Here's how the part is built. I have some questions about the finished solid (model axes, mm). A direction names the side the tool comes from. Coordinates: 2 decimals unless noted, no trailing zeros. Loops run counter-clockwise (first coordinate to the right, second up) from the corner with the lowest first, then second, coordinate; pieces in that order, holes last. Notation, with made-up numbers: M -11.75,41 L 9.25,41 A22 ccw 9.25,63 Z; hole C 54.5,-32 d8. An arc over 180 degrees is marked long. Use CSV: the item, a comma, the result in double quotes. Start each with the question number.
Q1. If we section it at D-D (z = 158.5): Please give me the cut outline in (x, y), and give its area (3 significant figures).
Q2. Please list where these lines run through material, in increasing order: probe 1 along Z at (x, y) = (193.5, -2.7); probe 2 along Z at (x, y) = (209, -2.05); probe 3 along Z at (x, y) = (421, -2.3). Write a range as [from, to].
Q3. If we section it at A-A (x = 37): Please give me the cut outline in (y, z).
Q4. If we section it at B-B (y = -2.35): State how many separate pieces and enclosed holes the cut face has, and give its area (3 significant figures).
Q5. Which directions (+Z, -Z, +X, -X, +Y, -Y) give clear straight access to the entire face, cutting with the end or side of a thin tool? Please do faces 5 (the flat face through (-7, 0, 118)), 6 (the cylindrical face through (-185.198, -1.479, -390.683)).
Q6. For pin 1 Ø0.9 at (x, y) = (429.5, -2) entering from +Z; pin 2 Ø0.5 at (x, y) = (-166.5, -1) entering from +Z; pin 3 Ø0.9 at (y, z) = (-1, 101.5) entering from +X, each with a flat end and sliding along its axis, tell me the tip position at first contact or that it passes through.
Q7. If we mould it in two halves opening along X, with no side actions, what happens to faces 1 (the cylindrical face through (-499.516, -1.479, 21.984)), 2 (the flat face through (-7, -3, 118)), 3 (the flat face through (-45.813, -1.479, 2.98)), 4 (the flat face through (356.448, -1.479, -3.983))? For each: +X half, -X half, draft (parallel to the pull), parting line (faces both ways), or undercut.
from build123d import *

# Parameters (mm, degrees)
F0_R     = 500
F0_W     = 23.0880718875
F0_H     = 198.6617711001
F1_DEPTH = 3


with BuildPart() as f1:
    # F0 (on Front) → F1 (new body)
    with BuildSketch(Plane.XZ):
        Circle(F0_R)
        with BuildLine():
            ThreePointArc((-274.567418569, -300.6351906095), (-305.6079419009, -166.1235155196), (-176.6063983823, -116.975711967))
            ThreePointArc((-176.6063983823, -116.975711967), (-123.1889327411, -95.6085057867), (-66.0571388124, -102.3865038656))
            ThreePointArc((-66.0571388124, -102.3865038656), (-40.8752164599, -88.187383642), (-13.1344654752, -80.0513549242))
            Line((-13.1344654752, -80.0513549242), (-13.1344654752, 41.8377829303))
            add(Edge.make_bspline(
                [(-13.1344654752, 41.8377829303), (-13.1344654752, 63.8388457836), (-11.2213295749, 89.6661804375)],
                knots=[0, 0, 0, 1, 1, 1], degree=2))
            Line((-11.2213295749, 89.6661804375), (-12.3083386092, 89.6661804375))
            Line((-12.3083386092, 89.6661804375), (-80.2681434307, -86.1684009433))
            Line((-80.2681434307, -86.1684009433), (-98.8777380971, -86.1684009433))
            Line((-98.8777380971, -86.1684009433), (-166.2722982207, 89.9270626057))
            Line((-166.2722982207, 89.9270626057), (-167.359307255, 89.9270626057))
            add(Edge.make_bspline(
                [(-167.359307255, 89.9270626057), (-165.4461713547, 69.0130087867), (-165.4461713547, 40.1855291983)],
                knots=[0, 0, 0, 1, 1, 1], degree=2))
            Line((-165.4461713547, 40.1855291983), (-165.4461713547, -86.1684009433))
            Line((-165.4461713547, -86.1684009433), (-186.7950287874, -86.1684009433))
            Line((-186.7950287874, -86.1684009433), (-186.7950287874, 112.4933701568))
            Line((-186.7950287874, 112.4933701568), (-152.0107396913, 112.4933701568))
            Line((-152.0107396913, 112.4933701568), (-89.0946567888, -51.3841118472))
            Line((-89.0946567888, -51.3841118472), (-88.0076477545, -51.3841118472))
            Line((-88.0076477545, -51.3841118472), (-24.5698005155, 112.4933701568))
            Line((-24.5698005155, 112.4933701568), (9.9536064123, 112.4933701568))
            Line((9.9536064123, 112.4933701568), (9.9536064123, -78.2026726688))
            ThreePointArc((9.9536064123, -78.2026726688), (53.773823289, -86.5372862236), (92.0090216607, -109.5100264977))
            ThreePointArc((92.0090216607, -109.5100264977), (168.8010036172, -106.3879816048), (230.8163361906, -151.7846134505))
            ThreePointArc((230.8163361906, -151.7846134505), (301.8959936917, -167.3086216291), (333.6679179608, -232.7598047248))
            ThreePointArc((333.6679179608, -232.7598047248), (303.4547141219, -296.9531582441), (234.7315185471, -314.581167554))
            ThreePointArc((234.7315185471, -314.581167554), (185.5253099789, -357.3835232893), (120.7398090278, -349.8914284782))
            ThreePointArc((120.7398090278, -349.8914284782), (38.3642732882, -404.4610167035), (-51.7318220906, -363.886856885))
            ThreePointArc((-51.7318220905, -363.886856885), (-58.6591581618, -362.0786424357), (-65.4384116096, -359.7766113262))
            ThreePointArc((-65.4384116096, -359.7766113262), (-186.9682580881, -390.1967718511), (-274.567418569, -300.6351906095))
        make_face(mode=Mode.SUBTRACT)
        Polygon((-357.1945649969, 91.9706395901), (-357.1945649969, -86.1684009433), (-380.2826368844, -86.1684009433), (-380.2826368844, 91.9706395901), (-443.198719787, 91.9706395901), (-443.198719787, 112.4933701568), (-294.2784820944, 112.4933701568), (-294.2784820944, 91.9706395901), align=None, mode=Mode.SUBTRACT)
        with Locations((-252.819957528, 13.1624846067)):
            Rectangle(F0_W, F0_H, mode=Mode.SUBTRACT)
        with BuildLine():
            add(Edge.make_bspline(
                [(212.8329725653, 88.4487303191), (236.877612403, 61.2735044628), (236.877612403, 13.4451069557)],
                knots=[0, 0, 0, 1, 1, 1], degree=2))
            add(Edge.make_bspline(
                [(236.877612403, 13.4451069557), (236.877612403, -34.2528494674), (212.7460118425, -61.5802565885)],
                knots=[0, 0, 0, 1, 1, 1], degree=2))
            add(Edge.make_bspline(
                [(212.7460118425, -61.5802565885), (188.6144112821, -88.9076637096), (145.6992946098, -88.9076637096)],
                knots=[0, 0, 0, 1, 1, 1], degree=2))
            add(Edge.make_bspline(
                [(145.6992946098, -88.9076637096), (101.8276099874, -88.9076637096), (77.9786317759, -62.0585405636)],
                knots=[0, 0, 0, 1, 1, 1], degree=2))
            add(Edge.make_bspline(
                [(77.9786317759, -62.0585405636), (54.1296535644, -35.2094174175), (54.1296535644, 13.7059891239)],
                knots=[0, 0, 0, 1, 1, 1], degree=2))
            add(Edge.make_bspline(
                [(54.1296535644, 13.7059891239), (54.1296535644, 62.2300724129), (78.0438523179, 88.9270142942)],
                knots=[0, 0, 0, 1, 1, 1], degree=2))
            add(Edge.make_bspline(
                [(78.0438523179, 88.9270142942), (101.9580510715, 115.6239561754), (145.9601767781, 115.6239561754)],
                knots=[0, 0, 0, 1, 1, 1], degree=2))
            add(Edge.make_bspline(
                [(145.9601767781, 115.6239561754), (188.7883327276, 115.6239561754), (212.8329725653, 88.4487303191)],
                knots=[0, 0, 0, 1, 1, 1], degree=2))
        make_face(mode=Mode.SUBTRACT)
        with BuildLine():
            Line((436.3220300077, 112.4933701568), (436.3220300077, -86.1684009433))
            Line((436.3220300077, -86.1684009433), (409.9729310174, -86.1684009433))
            Line((409.9729310174, -86.1684009433), (301.4024686762, 80.5353045497))
            Line((301.4024686762, 80.5353045497), (300.315459642, 80.5353045497))
            add(Edge.make_bspline(
                [(300.315459642, 80.5353045497), (302.4894777105, 51.1860606249), (302.4894777105, 26.7500975349)],
                knots=[0, 0, 0, 1, 1, 1], degree=2))
            Line((302.4894777105, 26.7500975349), (302.4894777105, -86.1684009433))
            Line((302.4894777105, -86.1684009433), (281.1406202777, -86.1684009433))
            Line((281.1406202777, -86.1684009433), (281.1406202777, 112.4933701568))
            Line((281.1406202777, 112.4933701568), (307.2288370998, 112.4933701568))
            Line((307.2288370998, 112.4933701568), (415.5384172728, -53.5581299157))
            Line((415.5384172728, -53.5581299157), (416.625426307, -53.5581299157))
            add(Edge.make_bspline(
                [(416.625426307, -53.5581299157), (416.3645441388, -49.9057795606), (415.4079761886, -29.9917740531)],
                knots=[0, 0, 0, 1, 1, 1], degree=2))
            add(Edge.make_bspline(
                [(415.4079761886, -29.9917740531), (414.4514082385, -10.0777685456), (414.7122904067, -1.5121373557)],
                knots=[0, 0, 0, 1, 1, 1], degree=2))
            Line((414.7122904067, -1.5121373557), (414.7122904067, 112.4933701568))
            Line((414.7122904067, 112.4933701568), (436.3220300077, 112.4933701568))
        make_face(mode=Mode.SUBTRACT)
    extrude(amount=F1_DEPTH)


solid = f1.part
Results below:
1,outline,"M -474.21,-3 L 474.21,-3 L 474.21,0 L -474.21,0 Z"
1,area,"2,850 mm^2"
2,probe 1,"[-461.04, -354.45], [-117.17, -77.39], [104.26, 461.04]"
2,probe 2,"[-454.22, -345.65], [-127.97, -65.55], [92.49, 454.22]"
2,probe 3,"[-269.74, -86.17], [112.49, 269.74]"
3,outline,"M -3,-498.63 L 0,-498.63 L 0,-404.56 L -3,-404.56 Z; M -3,-81.43 L 0,-81.43 L 0,498.63 L -3,498.63 Z"
4,separate pieces,"1"
4,enclosed holes,"5"
4,area,"556,000 mm^2"
5,face 5,"+Z, -Z, +X, -X, +Y"
5,face 6,"+Y, -Y"
6,pin 1,"z = 256.74"
6,pin 2,"z = 471.55"
6,pin 3,"x = 489.68"
7,face 1,"parting line"
7,face 2,"draft"
7,face 3,"undercut"
7,face 4,"undercut"
